from build123d import *

# Parameters (mm, degrees)
SKETCH_1_W          = 45
SKETCH_1_H          = 45
EXTRUDE_1_DEPTH     = 2
SKETCH_2_R          = 3.5
CUT_EXTRUDE_1_DEPTH = 32.882597134
EXTRUDE_START       = 0.5
SKETCH_3_R          = 13.5
SKETCH_3_R_2        = 3.5
EXTRUDE_2_DEPTH     = 0.5
SKETCH_4_R          = 1.5
CUT_EXTRUDE_4_DEPTH = 32.917863337
CHAMFER_1_SIZE      = 1


with BuildPart() as part:
    # 草图1 → 凸台-拉伸1 (new body)
    with BuildSketch(Plane(origin=(0, 0, 0), x_dir=(1, 0, 0), z_dir=(0, 1, 0))):
        Rectangle(SKETCH_1_W, SKETCH_1_H)
    extrude(amount=EXTRUDE_1_DEPTH)

    # 草图2 → 切除-拉伸1 (cut, through all)
    with BuildSketch(Plane(origin=(0, 2, 0), x_dir=(1, 0, 0), z_dir=(0, 1, 0))):
        with Locations(Location((0, 3, 0), (0, 0, 270))):
            Circle(SKETCH_2_R)
    extrude(amount=-CUT_EXTRUDE_1_DEPTH, mode=Mode.SUBTRACT)

    # 草图3 → 凸台-拉伸2 (add)
    with BuildSketch(Plane(origin=(0, 2, 0), x_dir=(1, 0, 0), z_dir=(0, 1, 0)).offset(EXTRUDE_START)):
        with Locations(Location((0, 3, 0), (0, 0, 270))):
            Circle(SKETCH_3_R)
        with Locations(Location((0, 3, 0), (0, 0, 270))):
            Circle(SKETCH_3_R_2, mode=Mode.SUBTRACT)
    extrude(amount=-EXTRUDE_2_DEPTH)

    # 草图4 → 切除-拉伸4 (cut, through all)
    with BuildSketch(Plane(origin=(0, 0, 0), x_dir=(1, 0, 0), z_dir=(0, 1, 0))):
        with Locations(Location((19.5, 19.5, 0), (0, 0, 90))):
            Circle(SKETCH_4_R)
        with Locations(Location((-19.5, 19.5, 0), (0, 0, 90))):
            Circle(SKETCH_4_R)
        with Locations(Location((-19.5, -19.5, 0), (0, 0, 90))):
            Circle(SKETCH_4_R)
        with Locations(Location((19.5, -19.5, 0), (0, 0, 90))):
            Circle(SKETCH_4_R)
    extrude(amount=CUT_EXTRUDE_4_DEPTH, mode=Mode.SUBTRACT)

    # 倒角1
    chamfer_1_edges = [part.edges().sort_by_distance(p)[0] for p in [
        (22.5, 1, 22.5),
        (-22.5, 1, 22.5),
        (-22.5, 1, -22.5),
        (22.5, 1, -22.5),
    ]]
    chamfer(chamfer_1_edges, length=CHAMFER_1_SIZE)


solid = part.part
Part model, mm, in its own coordinate system. A direction names the side the tool comes from. Give positions to 0.01 mm unless a question says otherwise; leave off trailing zeros. Loops run counter-clockwise (first coordinate to the right, second up) from the corner with the lowest first, then second, coordinate; pieces in that order, holes last. Notation, with made-up numbers: (3, 73) -> (38, 73) arc R19 cw to (38, 101) -> close; hole circle Ø11 at (31, 86). An arc over 180 degrees is marked (long way). Write each question's results on one line, items separated by ' | '. Start each with the question number.
Q1. Pin check, flat tips, straight feed: P1, Ø6, axis at x = 12, z = 15, coming from the -Y side; P2, Ø5, axis at x = 19.5, z = -19.5, coming from the +Y side. Stop position of each tip, or through.
Q2. Band-saw the part on B-B on x = 0. List the corners of the cut face in (y, z).
Q3. Band-saw the part on C-C on y = 1.3. List the corners of the cut face in (x, z).
Q4. Band-saw the part on A-A on x = -19.5. List the corners of the cut face in (y, z).
Q5. Wall check: L1, parallel to Z at x = 19.5, y = 0.9; L2, parallel to X at y = 0.8, z = -3. Give the ranges that are in metal, low to high.
Q6. Band-saw the part on D-D on z = 19.5. List the corners of the cut face in (x, y), plus the area to 3 significant figures.
Q7. Which spindle directions (+Z, -Z, +X, -X, +Y, -Y) get a long thin tool onto all of the face, cutting with end or side? Do faces 1 (the face through (5, 2, 10)), 2 (the face through (22.5, 1, 0)). Say none if no direction does.
Q8. Pull direction Z, two halves, no side cores. Call faces 3 (the face through (22, 1, -22)), 4 (the face through (0, 0, 5)), 5 (the face through (-20.51, 0.99, 20.61)): +Z half, -Z half, draft (parallel to the pull), parting line (faces both ways), or undercut.
Results are:
1) P1: stops at y = 0 | P2: stops at y = 2
2) outline: (0, -22.5) -> (2, -22.5) -> (2, -16.5) -> (2.5, -16.5) -> (2.5, -6.5) -> (0, -6.5) -> close; (0, 0.5) -> (2.5, 0.5) -> (2.5, 10.5) -> (2, 10.5) -> (2, 22.5) -> (0, 22.5) -> close
3) outline: (-22.5, -21.5) -> (-21.5, -22.5) -> (21.5, -22.5) -> (22.5, -21.5) -> (22.5, 21.5) -> (21.5, 22.5) -> (-21.5, 22.5) -> (-22.5, 21.5) -> close; hole circle Ø3 at (-19.5, -19.5); hole circle Ø3 at (-19.5, 19.5); hole circle Ø7 at (0, -3); hole circle Ø3 at (19.5, -19.5); hole circle Ø3 at (19.5, 19.5)
4) outline: (0, -22.5) -> (2, -22.5) -> (2, -21) -> (0, -21) -> close; (0, -18) -> (2, -18) -> (2, 18) -> (0, 18) -> close; (0, 21) -> (2, 21) -> (2, 22.5) -> (0, 22.5) -> close
5) L1: z = -22.5 to -21, -18 to 18, 21 to 22.5 | L2: x = -22.5 to -3.5, 3.5 to 22.5
6) outline: (-22.5, 0) -> (-21, 0) -> (-21, 2) -> (-22.5, 2) -> close; (-18, 0) -> (18, 0) -> (18, 2) -> (-18, 2) -> close; (21, 0) -> (22.5, 0) -> (22.5, 2) -> (21, 2) -> close | area: 78.0 mm²
7) face 1: +Y | face 2: +Z, -Z, +X, +Y, -Y
8) face 3: -Z half | face 4: draft | face 5: undercut
